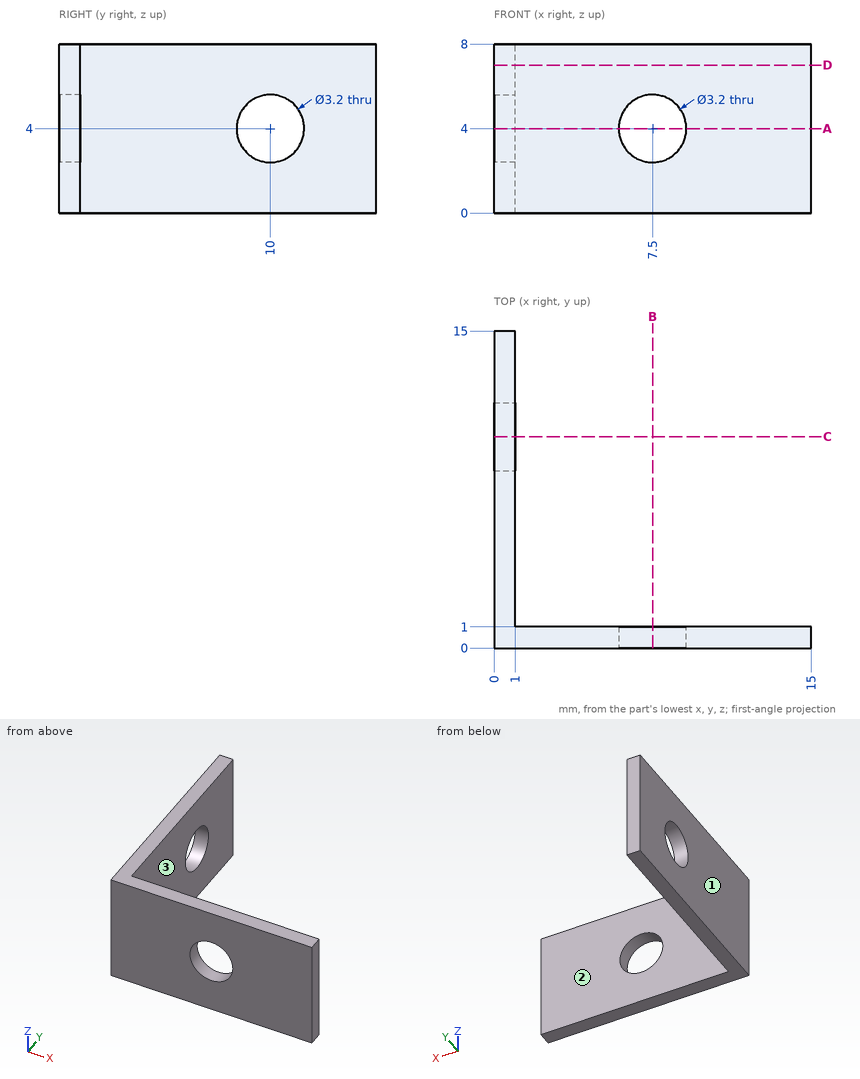
Design review of the part shown in the three views and the two pictorial views. Dimensions are in mm from the part's minimum x, y and z. Round coordinates to 2 decimals unless told otherwise and drop trailing zeros. Loops run counter-clockwise (first coordinate to the right, second up) from the corner with the lowest first, then second, coordinate; pieces in that order, holes last. Notation, with made-up numbers: (35.25, 69.25) -> (46.25, 69.25) arc R31 cw to (46.25, 97.25) -> close; hole circle Ø8 at (-8, 26.25). An arc over 180 degrees is marked (long way). Use one line per item in the form item = value. Start each with the question number.
Q1. We need section D-D on z = 7. Give the boundary of the cut face in (x, y), then the cut area to 3 significant figures.
Q2. We need section A-A on z = 4. Give the boundary of the cut face in (x, y).
Q3. Draft analysis for pull direction X (two halves, no side actions). For the marked faces 1, 2 and 3, state which applies: +X half, -X half, draft (parallel to the pull), parting line (faces both ways), or undercut.
Q4. For pin 1 Ø3 at (y, z) = (10, 4) entering from -X; pin 2 Ø2.5 at (y, z) = (6.5, 4.5) entering from +X, all flat-tipped, find the tip position at first contact; note any pin that passes through.
Q5. Wall thickness on line 1 along Z through (x, y) = (7.5, 0.35); line 2 along Y through (x, z) = (14, 3): over which ranges is each line inside the solid? List them lowest first. Write a range as [from, to].
Q6. We need section B-B on x = 7.5. Give the boundary of the cut face in (y, z).
Calculated:
q1.outline = (0, 0) -> (15, 0) -> (15, 1) -> (1, 1) -> (1, 15) -> (0, 15) -> close
q1.area = 29.0 mm²
q2.outline = (0, 0) -> (5.9, 0) -> (5.9, 1) -> (1, 1) -> (1, 8.4) -> (0, 8.4) -> close; (0, 11.6) -> (1, 11.6) -> (1, 15) -> (0, 15) -> close; (9.1, 0) -> (15, 0) -> (15, 1) -> (9.1, 1) -> close
q3.face_1 = -X half
q3.face_2 = draft
q3.face_3 = +X half
q4.pin_1 = through
q4.pin_2 = 1
q5.line_1 = [0, 2.4], [5.6, 8]
q5.line_2 = [0, 1]
q6.outline = (0, 0) -> (1, 0) -> (1, 2.4) -> (0, 2.4) -> close; (0, 5.6) -> (1, 5.6) -> (1, 8) -> (0, 8) -> close
